Geometry: final body of the model. Coordinates: model frame, mm. Face numbers are marked on the shaded views. Give positions to 0.01 mm unless a question says otherwise; leave off trailing zeros. Loops run counter-clockwise (first coordinate to the right, second up) from the corner with the lowest first, then second, coordinate; pieces in that order, holes last.
1. Section D-D, the plane y = 26. Output: boundary loops of the cut face in (x, z).
2. Draft query along Y for the marked faces 1, 2 and 3. Return one class per face: +Y half, -Y half, draft (parallel to the pull), parting line (faces both ways), or undercut.
3. Section C-C, the plane z = -3.5. Output: boundary loops of the cut face in (x, y), then the cut area to 3 significant figures.
4. Material intervals for line 1 along Y through (x, z) = (0, 4.75); line 2 along X through (y, z) = (0, 1.35); line 3 along Y through (x, z) = (0, 1.15), sorted ascending.
5. Section A-A, the plane x = 0. Output: boundary loops of the cut face in (y, z), then the cut area to 3 significant figures.
6. Section B-B, the plane y = 0. Output: boundary loops of the cut face in (x, z).
7. First-contact query: P1, Ø4, axis at x = 3.5, y = -3, coming from the -Z side; P2, Ø3, axis at x = -8.5, z = -3.5, coming from the +Y side; P3, Ø3, axis at y = 21, z = 1, coming from the -X side. Flat tips, straight axial feed; report the tip coordinate or a pass-through.
from build123d import *

# Parameters (mm, degrees)
SKETCH1_R           = 5
SKETCH1_R_2         = 2.75
BOSS_EXTRUDE1_DEPTH = 5
SKETCH2_W           = 3
SKETCH2_H           = 6.2
BOSS_EXTRUDE2_DEPTH = 5
FILLET1_R           = 1
FILLET2_R           = 5
CHAMFER1_SIZE       = 0.25


with BuildPart() as part:
    # Sketch1 → Boss-Extrude1 (new body)
    # profile 1 of 2: a face of its own
    with BuildSketch(Plane.XY):
        with Locations((0, 27)):
            Circle(SKETCH1_R)
    # profile 2 of 2: a face of its own
    with BuildSketch(Plane.XY):
        with BuildLine():
            Line((-4.811559492, 28.359740878), (-10, 10))
            Line((-10, 10), (-10, -10))
            Line((-10, -10), (10, -10))
            Line((10, -10), (10, 10))
            Line((10, 10), (4.811559492, 28.359740878))
            ThreePointArc((4.811559492, 28.359740878), (4.952665821, 27.686368174), (5, 27))
            ThreePointArc((5, 27), (-0.686368174, 22.047334179), (-4.811559492, 28.359740878))
        make_face()
        Circle(SKETCH1_R_2, mode=Mode.SUBTRACT)
    extrude(amount=BOSS_EXTRUDE1_DEPTH)

    # Sketch2 → Boss-Extrude2 (add)
    with BuildSketch(Plane(origin=(0, 0, 0), x_dir=(-1, 0, 0), z_dir=(0, 0, -1))):
        with Locations((-8.5, 0)):
            Rectangle(SKETCH2_W, SKETCH2_H)
        with Locations((8.5, 0)):
            Rectangle(SKETCH2_W, SKETCH2_H)
    extrude(amount=BOSS_EXTRUDE2_DEPTH)

    # Fillet1
    fillet1_edges = [part.edges().sort_by_distance(p)[0] for p in [
        (10, -10, 2.5),
        (-10, -10, 2.5),
        (7, 0, 0),
        (-7, 0, 0),
    ]]
    fillet(fillet1_edges, radius=FILLET1_R)

    # Fillet2
    fillet2_edges = [part.edges().sort_by_distance(p)[0] for p in [
        (10, 10, 2.5),
        (-10, 10, 2.5),
    ]]
    fillet(fillet2_edges, radius=FILLET2_R)

    # Sketch4 → CSK for M5 Flat Head Machine Screw1 (revolve, cut)
    with BuildSketch(Plane(origin=(0, 0, 5), x_dir=(0, -1, 0), z_dir=(1, 0, 0))):
        Polygon((0, 0), (0, 10), (2.75, 10), (2.75, 2.75), (5, 0.5), (5, 0), align=None)
    revolve(axis=Axis((0, 0, 11.35), (0, 0, -1)), mode=Mode.SUBTRACT)

    # Chamfer1
    chamfer1_edges = [part.edges().sort_by_distance(p)[0] for p in [
        (-10, 6.203535995, 0),
        (-7.311559492, 19.513276873, 0),
        (10, 6.203535995, 0),
        (-9.952665821, 9.993440164, 0),
        (9.952665821, 9.993440164, 0),
        (10, 0.153535995, 5),
        (-7.311559492, 19.513276873, 5),
        (-10, 0.153535995, 5),
        (-9.952665821, 9.993440164, 5),
        (9.952665821, 9.993440164, 5),
        (0, 32, 0),
        (10, -6.05, 0),
        (-10, -6.05, 0),
        (10, 0, -5),
        (8.5, -3.1, -5),
        (7, 0, -5),
        (8.5, 3.1, -5),
        (-7, 0, -5),
        (-8.5, -3.1, -5),
        (-10, 0, -5),
        (-8.5, 3.1, -5),
        (0, -10, 0),
        (-9.707106781, -9.707106781, 0),
        (9.707106781, -9.707106781, 0),
        (0, -10, 5),
        (0, 32, 5),
        (-9.707106781, -9.707106781, 5),
        (9.707106781, -9.707106781, 5),
        (7.311559492, 19.513276873, 0),
        (7.311559492, 19.513276873, 5),
    ]]
    chamfer(chamfer1_edges, length=CHAMFER1_SIZE)


solid = part.part
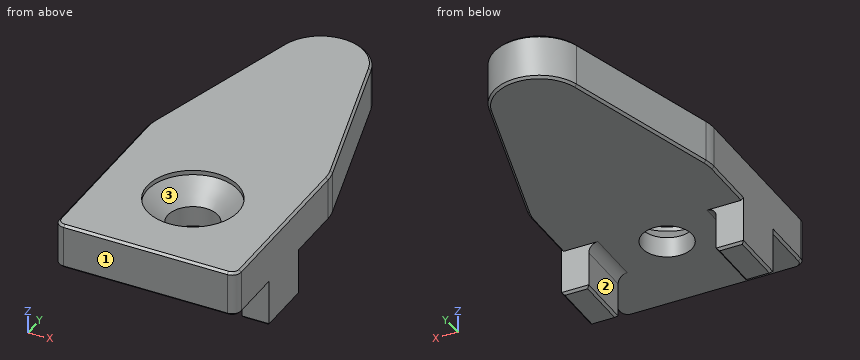
Answers below:
1. outline: (-5.48, 0.25) - (-5.22, 0) - (5.22, 0) - (5.48, 0.25) - (5.48, 4.75) - (5.22, 5) - (-5.22, 5) - (-5.48, 4.75) - close
2. face 1: -Y half
2. face 2: draft
2. face 3: undercut
3. outline: (-10, -3.1) - (-7, -3.1) - (-7, 3.1) - (-10, 3.1) - close; (7, -3.1) - (10, -3.1) - (10, 3.1) - (7, 3.1) - close
3. area: 37.2 mm2
4. line 1: y = -10 to -5, 5 to 32
4. line 2: x = -10 to -2.75, 2.75 to 10
4. line 3: y = -10 to -2.75, 2.75 to 32
5. outline: (-10, 0.25) - (-9.75, 0) - (-2.75, 0) - (-2.75, 2.25) - (-5, 4.5) - (-5, 5) - (-9.75, 5) - (-10, 4.75) - close; (2.75, 0) - (31.75, 0) - (32, 0.25) - (32, 4.75) - (31.75, 5) - (5, 5) - (5, 4.5) - (2.75, 2.25) - close
5. area: 175 mm2
6. outline: (-10, -4.75) - (-9.75, -5) - (-7.25, -5) - (-7, -4.75) - (-7, -1) arc R1 cw to (-6, 0) - (-2.75, 0) - (-2.75, 2.25) - (-5, 4.5) - (-5, 5) - (-9.75, 5) - (-10, 4.75) - close; (2.75, 0) - (6, 0) arc R1 cw to (7, -1) - (7, -4.75) - (7.25, -5) - (9.75, -5) - (10, -4.75) - (10, 4.75) - (9.75, 5) - (5, 5) - (5, 4.5) - (2.75, 2.25) - close
7. P1: stops at z = 0
7. P2: stops at y = 3.1
7. P3: stops at x = -7.32
